from build123d import *

# Parameters (mm, degrees)
F0_W     = 35.56
F0_H     = 162.057699
F2_R     = 5.969
F3_DEPTH = 22.86
F4_R     = 6.096
F5_DEPTH = 25.4


with BuildPart() as f1:
    # F0 (on Front) → F1 (revolve)
    with BuildSketch(Plane.XZ):
        with Locations((-17.78, 5.673615)):
            Rectangle(F0_W, F0_H)
    revolve(axis=Axis((0, 0, 4.235234), (0, 0, -1)))

    # F2 (on face) → F3 (join)
    with BuildSketch(Plane(origin=(0, 0, -75.355234), x_dir=(1, 0, 0), z_dir=(0, 0, -1))):
        Circle(F2_R)
    extrude(amount=F3_DEPTH)

    # F4 (on face) → F5 (cut)
    with BuildSketch(Plane.XY.offset(86.702465)):
        Circle(F4_R)
    extrude(amount=-F5_DEPTH, mode=Mode.SUBTRACT)


solid = f1.part
Design review of the part built by this model. Coordinates are the model's own, in mm. A direction names the side the tool comes from. Coordinates: 2 decimals unless noted, no trailing zeros. Order: outer loops, then holes, each group sorted by start corner. A loop starts at its lowest first (then second) coordinate and runs counter-clockwise, first axis right, second up.
Item 1: Take a section at C-C, the plane z = -30.5. Write out the cut boundary in (x, y).
Item 2: Take a section at D-D, the plane x = 19.5. Write out the cut boundary in (y, z).
Item 3: For pin 1 Ø11 at (x, y) = (0, 0) entering from +Z; pin 2 Ø21.5 at (x, y) = (16, -5.5) entering from -Z; pin 3 Ø10 at (x, z) = (15, 40) entering from +Y (3 decimals), all flat-tipped, find the tip position at first contact; note any pin that passes through.
Item 4: Take a section at A-A, the plane x = 0. Write out the cut boundary in (y, z), then the cut area to 3 significant figures.
Item 5: The part is to be moulded in two halves that separate along Y. For faces 1 (the cylindrical face through (-1.294, 5.827, -86.625)), 2 (the flat face through (0, -7, 86.702)), 3 (the flat face through (0, 0, 61.302)), say which applies: pulls with the +Y half, pulls with the -Y half, needs draft (parallel to the pull), parting line crosses it, or undercut.
Item 6: For line 1 (Y direction, x = 0, z = 77.5); line 2 (Z direction, x = 24, y = 21.5); line 3 (X direction, y = -2, z = 64), list the stretches that pass through material, from the lowest coordinate up.
Item 7: For faces 4 (the cylindrical face through (7.709, -34.714, 6.808)), 5 (the cylindrical face through (-0.794, 6.044, 74.18)), list the 3-axis set-ups (+Z, -Z, +X, -X, +Y, -Y) from which the entire face can be reached by the end or side of a thin tool; tool diameter is ignored.
The answers:
1. outline: circle Ø71.12 at (0, 0)
2. outline: (-29.74, -75.36) - (29.74, -75.36) - (29.74, 86.7) - (-29.74, 86.7) - close
3. pin 1: stops at z = 61.3
3. pin 2: stops at z = -75.36
3. pin 3: stops at y = 34.125
4. outline: (-35.56, -75.36) - (-5.97, -75.36) - (-5.97, -98.22) - (5.97, -98.22) - (5.97, -75.36) - (35.56, -75.36) - (35.56, 86.7) - (6.1, 86.7) - (6.1, 61.3) - (-6.1, 61.3) - (-6.1, 86.7) - (-35.56, 86.7) - close
4. area: 11,500 mm2
5. face 1: parting line crosses it
5. face 2: needs draft
5. face 3: undercut
6. line 1: y = -35.56 to -6.1, 6.1 to 35.56
6. line 2: z = -75.36 to 86.7
6. line 3: x = -35.5 to -5.76, 5.76 to 35.5
7. face 4: +Z, -Z
7. face 5: +Z
